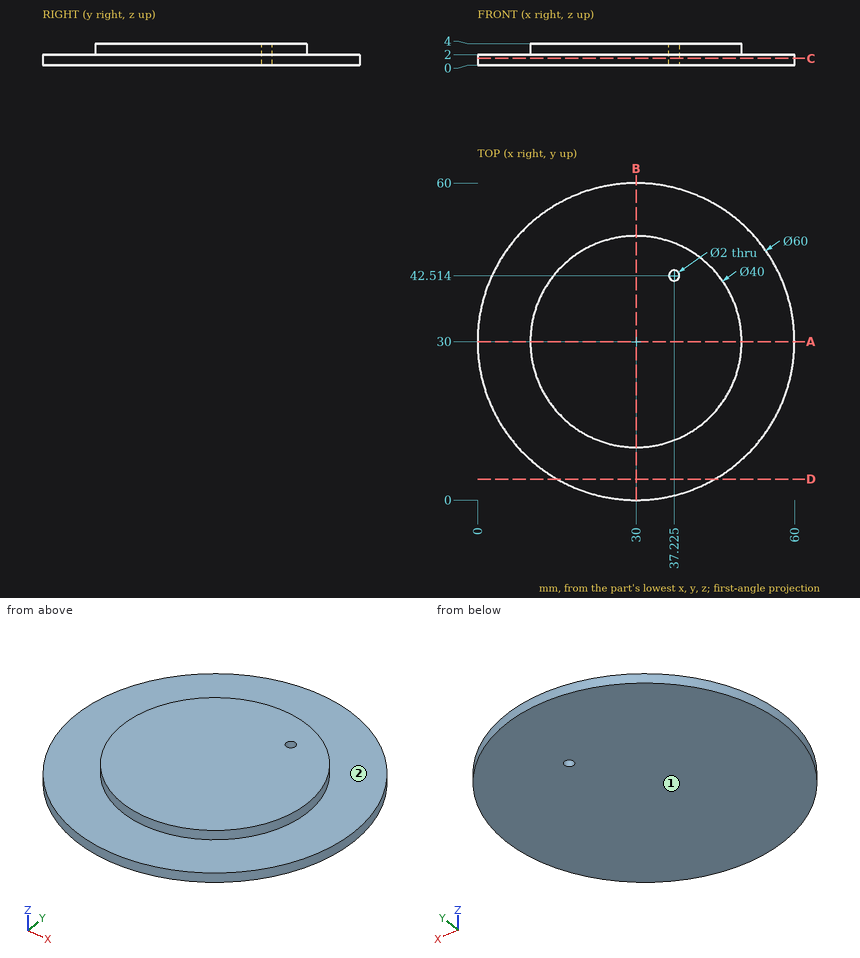
The figure shows three views and two pictorial views of one solid part (mm, origin at its lowest corner). Answer the questions. A direction names the side the tool comes from. Give positions to 0.01 mm unless a question says otherwise; leave off trailing zeros. Write each loop counter-clockwise with the first axis right and the second up, starting at its lowest first coordinate (ties: lowest second). Pieces come first, ordered by that corner, then holes.
Q1. Given pin 1 (2.5 mm diameter, centred on x = 37.23, y = 42.51, fed in from -Z); pin 2 (1.5 mm diameter, centred on y = 39.5, z = 2.5, fed in from -X); pin 3 (10 mm diameter, centred on x = 6, y = 52.5, fed in from +Z), each flat-ended and moving along its own axis, determine where each tip first touches the part or whether it passes through.
Answer:
pin 1: stops at z = 0
pin 2: stops at x = 1.36
pin 3: stops at z = 2
Q2. The part is cut by section A-A on y = 30. Give the vertices of the cut face in (x, z), and give its area (3 significant figures).
Answer:
outline: (0, 0) - (60, 0) - (60, 2) - (50, 2) - (50, 4) - (10, 4) - (10, 2) - (0, 2) - close
area: 200 mm2
Q3. The part is cut by section D-D on y = 4. Give the vertices of the cut face in (x, z).
Answer:
outline: (15.03, 0) - (44.97, 0) - (44.97, 2) - (15.03, 2) - close
Q4. The part is cut by section C-C on z = 1.3. Give the vertices of the cut face in (x, y) (1 decimal), and give its area (3 significant figures).
Answer:
outline: circle Ø60 at (30, 30); hole circle Ø2 at (37.2, 42.5)
area: 2,820 mm2
Q5. A tool of negligible diameter and unlimited length cuts with its end or side. For the marked faces 1 and 2, from which of +Z, -Z, +X, -X, +Y, -Y can it reach the whole face along a straight path? Write none if from no direction.
Answer:
face 1: -Z, +X, -X, +Y, -Y
face 2: +Z
Q6. Straight lines are drawn through the part: L1, parallel to Z at x = 37, y = 52; L2, parallel to X at y = 29.5, z = 1.9; L3, parallel to Y at x = 36.5, z = 1.7 (1 decimal). For each, find the intervals that lie inside material, in ascending order.
Answer:
L1: z = 0 to 2
L2: x = 0 to 60
L3: y = 0.7 to 41.8, 43.2 to 59.3
